The listing builds one solid part. Answer for the finished solid, in the listing's coordinates (mm). Face numbers are marked on the shaded views. A direction names the side the tool comes from. Coordinates: 2 decimals unless noted, no trailing zeros. Answer as a JSON object with one key per item and string values. Group by question number.
1. Determine the mould class of the marked faces 1, 2 and 3 for opening direction Z: released by +Z, released by -Z, zero draft, split by the parting line, or undercut.
2. A cutting plane is placed at A-A on x = 18. State how many separate pieces and enclosed holes the cut face has, and give its area (3 significant figures).
3. Straight lines are drawn through the part: L1, parallel to Z at x = 14, y = 32; L2, parallel to Y at x = 13.5, z = 7.5; L3, parallel to Y at x = 17, z = 59. For each, find the intervals that lie inside material, in ascending order.
4. Given pin 1 (4 mm diameter, centred on x = 21, y = 44, fed in from +Z); pin 2 (6 mm diameter, centred on x = 23, z = -51.5, fed in from +Y); pin 3 (11 mm diameter, centred on y = 59, z = 1.5, fed in from -X); pin 4 (10.5 mm diameter, centred on y = -31.5, z = -32.5, fed in from -X), each flat-ended and moving along its own axis, determine where each tip first touches the part or whether it passes through.
5. For the marked faces 4, 5 and 6, determine the directions among +Z, -Z, +X, -X, +Y, -Y from which every point of the face is accessible in a straight line to the end or side of a thin tool.
from build123d import *

# Parameters (mm, degrees)
SKETCH1_R                = 101.6
SKETCH1_R_2              = 76.2
BOSS_EXTRUDE1_DEPTH      = 38.1
FILLET1_R                = 6.35
SKETCH2_R                = 25.4
BOSS_EXTRUDE2_DEPTH      = 12.7
BOSS_EXTRUDE2_DEPTH_BACK = 12.7
SKETCH3_W                = 10.17723869
SKETCH3_H                = 65.923797021
BOSS_EXTRUDE3_DEPTH      = 6.35
BOSS_EXTRUDE3_DEPTH_BACK = 6.35


with BuildPart() as part:
    # Sketch1 → Boss-Extrude1 (new body)
    with BuildSketch(Plane(origin=(0, 0, 0), x_dir=(0, 0, -1), z_dir=(1, 0, 0))):
        Circle(SKETCH1_R)
        Circle(SKETCH1_R_2, mode=Mode.SUBTRACT)
    extrude(amount=BOSS_EXTRUDE1_DEPTH)

    # Fillet1
    fillet1_edges = [part.edges().sort_by_distance(p)[0] for p in [
        (0, 0, 101.6),
        (38.1, 0, 101.6),
    ]]
    fillet(fillet1_edges, radius=FILLET1_R)



with BuildPart() as body_2:
    # Sketch2 → Boss-Extrude2 (new body, two sides)
    with BuildSketch(Plane.ZY.offset(-19.05)) as boss_extrude2_sk:
        Circle(SKETCH2_R)
        Polygon((-5.356755209, -5.00684601), (1.657678233, -7.142509098), (7.014433442, -2.135663088), (5.356755209, 5.00684601), (-1.657678233, 7.142509098), (-7.014433442, 2.135663088), align=None, mode=Mode.SUBTRACT)
    extrude(amount=BOSS_EXTRUDE2_DEPTH)
    extrude(boss_extrude2_sk.sketch, amount=-BOSS_EXTRUDE2_DEPTH_BACK)


with BuildPart() as part_1:
    add(part.part)

    add(body_2.part)  # Boss-Extrude3 merges body 2
    # Sketch3 → Boss-Extrude3 (add, two sides)
    with BuildSketch(Plane.ZY.offset(-19.05)) as boss_extrude3_sk:
        Polygon((6.933069311, 9.87864093), (12.021688656, 1.064893684), (69.11337159, 34.026792195), (64.024752245, 42.840539441), align=None)
        with Locations((0, 43.905433126)):
            Rectangle(SKETCH3_W, SKETCH3_H)
        Polygon((12.021688656, -1.064893684), (6.933069311, -9.87864093), (64.024752245, -42.840539441), (69.11337159, -34.026792195), align=None)
        with Locations((0, -43.905433126)):
            Rectangle(SKETCH3_W, SKETCH3_H)
        Polygon((-6.933069311, -9.87864093), (-12.021688656, -1.064893684), (-69.11337159, -34.026792195), (-64.024752245, -42.840539441), align=None)
        Polygon((-12.021688656, 1.064893684), (-6.933069311, 9.87864093), (-64.024752245, 42.840539441), (-69.11337159, 34.026792195), align=None)
    extrude(amount=BOSS_EXTRUDE3_DEPTH)
    extrude(boss_extrude3_sk.sketch, amount=-BOSS_EXTRUDE3_DEPTH_BACK)


solid = part_1.part
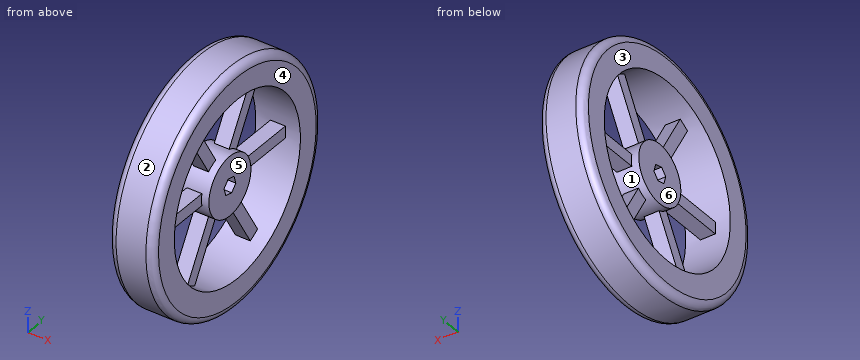
From the geometry:
{
 "1": {"face 1": "undercut", "face 2": "split by the parting line", "face 3": "zero draft"},
 "2": {"separate pieces": "1", "enclosed holes": "7", "area": "19,200 mm²"},
 "3": {"L1": "z = -96.43 to -69.16, -65.6 to -45.25, -5.09 to 5.09, 45.25 to 65.6, 69.16 to 96.43", "L2": "y = -101.32 to -75.83, -24.27 to 24.27, 75.83 to 101.32", "L3": "y = -82.71 to -48.22, -39.94 to -28.19, 28.19 to 39.94, 48.22 to 82.71"},
 "4": {"pin 1": "stops at z = 92.51", "pin 2": "stops at y = 89.28", "pin 3": "stops at x = 12.7", "pin 4": "passes through"},
 "5": {"face 4": "+Z, -Z, +X, +Y, -Y", "face 5": "+X", "face 6": "-X"}
}
